from build123d import *

# Parameters (mm, degrees)
F0_R     = 30
F0_R_2   = 10
F1_DEPTH = 65
F2_R     = 9.99999


# Not quite as in the source:
# - a fillet or chamfer is up to 0.001 mm smaller than in the source, because OpenCascade refuses the exact size


with BuildPart() as f1:
    # F0 (on Right) → F1 (new body)
    with BuildSketch(Plane.YZ):
        Circle(F0_R)
        Circle(F0_R_2, mode=Mode.SUBTRACT)
    extrude(amount=F1_DEPTH)

    # F2 (radius 10 in the source; OpenCascade refuses exactly that, so slightly less here)
    f2_edges = [f1.edges().sort_by_distance(p)[0] for p in [
        (65, -30, 0),
        (65, -10, 0),
        (32.5, 30, 0),
        (0, -30, 0),
        (0, -10, 0),
        (32.5, 10, 0),
    ]]
    fillet(f2_edges, radius=F2_R)


solid = f1.part
For this review, take the finished solid that the model builds, in its own axes (mm). Give positions to 0.01 mm unless a question says otherwise; leave off trailing zeros. Loops run counter-clockwise (first coordinate to the right, second up) from the corner with the lowest first, then second, coordinate; pieces in that order, holes last. Notation, with made-up numbers: M -14.5,64 L 3.5,64 A20 ccw 3.5,99 Z; hole C -6,48 d5. An arc over 180 degrees is marked long. Answer as a JSON object with one key per item and string values. Group by question number.
Q1. Add section C-C on x = 14. Give the boundary of the cut face in (y, z), and give its area (3 significant figures).
Q2. Mouldability with a two-part tool opening along Z and no side actions: class faces 1 (the cylindrical face through (32.18, -2.17, -9.76)), 2 (the cylindrical face through (32.18, -29.97, 1.32)) as +Z half, -Z half, draft (parallel to the pull), parting line (faces both ways), or undercut.
Q3. For probe 1 along Z at (x, y) = (34.5, 0); probe 2 along Y at (x, z) = (20.5, -7); probe 3 along Y at (x, z) = (11.5, 3.5), list the stretches that pass through material, from the lowest coordinate up. Write a range as [from, to].
Q4. Insertion check: P1, Ø8, axis at x = 29, y = 11, coming from the -Z side; P2, Ø12, axis at y = 16.5, z = -21.5, coming from the +X side; P3, Ø8, axis at y = -19, z = -22, coming from the -X side. Each pin has a flat end and moves straight along its axis. Give the tip position at first contact, or say it passes through.
Checked values:
{
 "1": {"outline": "C 0,0 d60; hole C 0,0 d20", "area": "2,510 mm²"},
 "2": {"face 1": "undercut", "face 2": "parting line"},
 "3": {"probe 1": "[-30, -10], [10, 30]", "probe 2": "[-29.17, -7.14], [7.14, 29.17]", "probe 3": "[-29.8, -9.37], [9.37, 29.8]"},
 "4": {"P1": "z = -29.17", "P2": "x = 64.94", "P3": "x = 1.38"}
}
